from build123d import *

# Parameters (mm, degrees)
BOSS_EXTRUDE2_DEPTH                      = 9.5
CBORE_FOR_M12_HEX_HEAD_BOLT2_D           = 6.75
CBORE_FOR_M12_HEX_HEAD_BOLT2_CBORE_D     = 25
CBORE_FOR_M12_HEX_HEAD_BOLT2_CBORE_DEPTH = 5


with BuildPart() as part:
    # Sketch1 → Boss-Extrude2 (new, symmetric)
    with BuildSketch(Plane(origin=(0, 0, 0), x_dir=(1, 0, 0), z_dir=(0, 1, 0))):
        with BuildLine():
            ThreePointArc((-12.7, 0), (0, 12.7), (12.7, 0))
            Line((12.7, 0), (25.09, 0))
            Line((25.09, 0), (25.09, 19))
            Line((25.09, 19), (-25.09, 19))
            Line((-25.09, 19), (-25.09, 0))
            Line((-25.09, 0), (-12.7, 0))
        make_face()
    extrude(amount=BOSS_EXTRUDE2_DEPTH, both=True)

    # CBORE for M12 Hex Head Bolt2 (through all)
    with Locations(Plane(origin=(18.889837659, -0.028068109, -19), x_dir=(-1, 0, 0), z_dir=(0, 0, -1))):
        with Locations((0, 0), (37.835811537, -0.112272438)):
            CounterBoreHole(CBORE_FOR_M12_HEX_HEAD_BOLT2_D / 2, CBORE_FOR_M12_HEX_HEAD_BOLT2_CBORE_D / 2, CBORE_FOR_M12_HEX_HEAD_BOLT2_CBORE_DEPTH)


solid = part.part
Here's how the part is built. I have some questions about the finished solid (model axes, mm). A direction names the side the tool comes from. Give positions to 0.01 mm unless a question says otherwise; leave off trailing zeros. Order: outer loops, then holes, each group sorted by start corner. A loop starts at its lowest first (then second) coordinate and runs counter-clockwise, first axis right, second up. Notation, with made-up numbers: (17, -15.5) -> (66, -15.5) arc R24 cw to (66, 5.5) -> close; hole circle Ø3 at (-7, -4.5). An arc over 180 degrees is marked (long way). Use a Markdown table: item, result. Add a question column.
Item 1: Imagine slicing it at B-B on x = -17. Please give me the cut outline in (y, z), plus the area to 3 significant figures.
Item 2: Will these pins go through, and if not, where does the flat tip stop? pin 1 (5 mm diameter, centred on y = -5.5, z = -17, fed in from -X); pin 2 (5.5 mm diameter, centred on x = -16.5, y = 1, fed in from -Z).
Item 3: If we mould it in two halves opening along Y, with no side actions, what happens to faces 4 (the face through (0, 9.5, -14)), 5 (the face through (-6.45, 0.23, -16.54)), 6 (the face through (-0.279, 0.133, -12.697))? For each: pulls with the +Y half, pulls with the -Y half, needs draft (parallel to the pull), parting line crosses it, or undercut.
Item 4: For faces 1 (the face through (0, -9.5, -14)), 2 (the face through (-16, 2, -14)), 3 (the face through (15.9, -2, -14)), which set-ups out of +Z, -Z, +X, -X, +Y, -Y let a thin tool reach every point of the face, with its end or its side?
Item 5: Imagine slicing it at A-A on z = -7.75. Please give me the cut outline in (x, y) (3 decimals), plus the area to 3 significant figures.
Item 6: I need wall thicknesses on line 1 (X direction, y = -2.5, z = -11.5); line 2 (X direction, y = -1.25, z = -9.75); line 3 (Z direction, x = 22, y = 1.5). Which ranges of each line are inside material? Lowest first, please.
Item 7: Imagine slicing it at D-D on y = 5.75. Please give me the cut outline in (x, z).
Item 8: Imagine slicing it at C-C on z = -2.5. Give the number of separate pieces and of enclosed holes in the cut face, plus the area to 3 significant figures.
Data:
| question | item | result |
|---|---|---|
| 1 | outline | (-9.5, -14) -> (-2.9, -14) -> (-2.9, 0) -> (-9.5, 0) -> close; (2.62, -14) -> (9.5, -14) -> (9.5, 0) -> (2.62, 0) -> close |
| 1 | area | 189 mm² |
| 2 | pin 1 | stops at x = -9.23 |
| 2 | pin 2 | stops at z = -14 |
| 3 | face 4 | pulls with the +Y half |
| 3 | face 5 | undercut |
| 3 | face 6 | needs draft |
| 4 | face 1 | +Z, -Z, +X, -X, -Y |
| 4 | face 2 | -Z, -X |
| 4 | face 3 | -Z, +X |
| 5 | outline | (-25.09, -9.5) -> (-10.061, -9.5) -> (-10.061, 9.5) -> (-25.09, 9.5) -> close; (10.061, -9.5) -> (25.09, -9.5) -> (25.09, 9.5) -> (10.061, 9.5) -> close; hole circle Ø6.75 at (-18.946, -0.14); hole circle Ø6.75 at (18.89, -0.028) |
| 5 | area | 500 mm² |
| 6 | line 1 | x = -25.09 to -21.36, -16.53 to -5.39, 5.39 to 16.59, 21.19 to 25.09 |
| 6 | line 2 | x = -25.09 to -22.13, -15.76 to -8.14, 8.14 to 15.74, 22.04 to 25.09 |
| 6 | line 3 | z = -14 to 0 |
| 7 | outline | (-25.09, -14) -> (-7.92, -14) -> (-7.92, -19) -> (7.81, -19) -> (7.81, -14) -> (25.09, -14) -> (25.09, 0) -> (12.7, 0) arc R12.7 cw to (-12.7, 0) -> (-25.09, 0) -> close |
| 8 | separate pieces | 2 |
| 8 | enclosed holes | 2 |
| 8 | area | 409 mm² |
